Autodesk Inventor part; units mm, degrees
ref_plane "YZ Plane" through (0, 0, 0) normal (1, 0, 0) x (0, 1, 0)
ref_plane "XZ Plane" through (0, 0, 0) normal (0, 1, 0) x (-1, 0, 0)
ref_plane "XY Plane" through (0, 0, 0) normal (0, 0, 1) x (1, 0, 0)
sketch "Sketch1" plane through (0, 0, 0) normal (0, 0, 1) x (1, 0, 0)
  circle A0 centre (0, 0) radius 10
  circle A1 centre (0, 0) radius 8
  dimension "d0" = 20
  dimension "d1" = 2
extrude "Extrusion1" add sketch "Sketch1" along normal blind 115
sketch "Sketch2" plane through (0, 0, 0) normal (0, 0, -1) x (-1, 0, 0)
  circle A0 centre (0, 0) radius 16.5
  circle A1 centre (0, 0) radius 8
  circle A2 centre (0, 0) radius 8 construction
  dimension "d4" = 33
extrude "Extrusion2" add sketch "Sketch2" against normal blind 3
sketch "Sketch3" plane through (0, 0, 3) normal (0, 0, 1) x (1, 0, 0)
  circle A0 centre (9.8995, 9.8995) radius 1.55
  line L0 (9.8995, 9.8995) -> (0, 0) construction
  line L1 (0, 0) -> (4.9931, 0) construction
  dimension "d7" = 14
  dimension "d8" = 3.1
  dimension "d14" = 45
extrude "Extrusion3" cut sketch "Sketch3" against normal through all
sketch "Sketch7" plane through (0, 0, 3) normal (0, 0, 1) x (1, 0, 0)
  circle A0 centre (0, 0) radius 11
  circle A1 centre (0, 0) radius 10
  circle A2 centre (0, 0) radius 10 construction
  dimension "d30" = 1
extrude "Extrusion7" add sketch "Sketch7" along normal blind 2
pattern_circular "Circular Pattern1" count 4 over 360 about axis through (0, 0, 0) along (0, 0, 1) of "Extrusion3"
sketch "Sketch5" plane through (0, 0, 3) normal (0, 0, 1) x (1, 0, 0)
  line L0 (-0.5, 10) -> (0.5, 10)
  line L1 (0.5, 10) -> (0.5, 20)
  line L2 (0.5, 20) -> (-0.5, 20)
  line L3 (-0.5, 20) -> (-0.5, 10)
  line L4 (-0.5, 10) -> (0.5, 20) construction
  line L5 (0.5, 10) -> (-0.5, 20) construction
  point P0 (0, 0)
  point P1 (0, 15)
  point P2 (0, 15)
  dimension "d21" = 1
  dimension "d22" = 10
  dimension "d23" = 10
extrude "Extrusion5" cut sketch "Sketch5" along normal blind 2 and the other way blind 2
sketch "Sketch6" plane through (0, 0, 0) normal (0, 1, 0) x (-1, 0, 0)
  circle A0 centre (0, 112) radius 1.25
  line L0 (10, 115) -> (-10, 115) construction
  point P0 (0, 0)
  dimension "d26" = 3
  dimension "d27" = 2.5
extrude "Extrusion6" cut sketch "Sketch6" along normal through all both and the other way through all
properties part number "Coil_Stand"
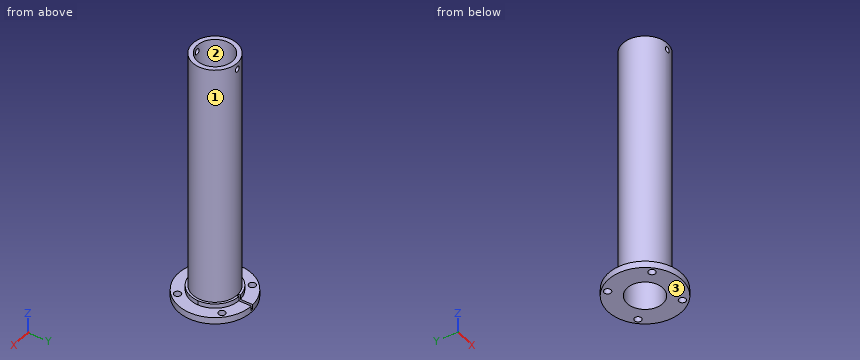
Check sheet for the modelled part. Datum: model origin and axes. Units: mm. Face numbers are marked on the shaded views. Round coordinates to 2 decimals unless told otherwise and drop trailing zeros. Write each loop counter-clockwise with the first axis right and the second up, starting at its lowest first coordinate (ties: lowest second). Pieces come first, ordered by that corner, then holes. Notation, with made-up numbers: (54, 60) -> (81, 60) arc R25 ccw to (81, 74) -> close; hole circle Ø8 at (30, 41). An arc over 180 degrees is marked (long way). Put each result on its own line as item: value.
(1) Sectioned sample at C-C (y = -2). Enter the section's corners in (x, z), plus the area to 3 significant figures.
Values found:
outline: (-16.38, 0) -> (-7.75, 0) -> (-7.75, 115) -> (-9.8, 115) -> (-9.8, 5) -> (-10.82, 5) -> (-10.82, 3) -> (-16.38, 3) -> close; (7.75, 0) -> (16.38, 0) -> (16.38, 3) -> (10.82, 3) -> (10.82, 5) -> (9.8, 5) -> (9.8, 115) -> (7.75, 115) -> close
area: 516 mm^2
(2) Mould release check, pull along Y, two halves, no side actions. Record for the marked faces 1, 2 and 3: released by +Y, released by -Y, zero draft, split by the parting line, or undercut.
Values found:
face 1: split by the parting line
face 2: undercut
face 3: zero draft
(3) Go/stop test with flat-tipped pins: pin 1 Ø3 at (x, z) = (0, 112) entering from -Y; pin 2 Ø10 at (y, z) = (-2, 63.5) entering from +X; pin 3 Ø0.5 at (x, z) = (0, 4) entering from +Y; pin 4 Ø6.5 at (x, y) = (0, 3.5) entering from +Z. Record where each tip stops, or that it passes through.
Values found:
pin 1: stops at y = -10
pin 2: stops at x = 10
pin 3: stops at y = 10
pin 4: passes through
(4) Sectioned sample at A-A (x = -6). Enter the section's corners in (y, z).
Values found:
outline: (-15.37, 0) -> (-5.29, 0) -> (-5.29, 115) -> (-8, 115) -> (-8, 5) -> (-9.22, 5) -> (-9.22, 3) -> (-15.37, 3) -> close; (5.29, 0) -> (15.37, 0) -> (15.37, 3) -> (9.22, 3) -> (9.22, 5) -> (8, 5) -> (8, 115) -> (5.29, 115) -> close
(5) Sectioned sample at B-B (z = 105). Enter the section's corners in (x, y), plus the area to 3 significant figures.
Values found:
outline: circle Ø20 at (0, 0); hole circle Ø16 at (0, 0)
area: 113 mm^2
(6) Material ranges on line 1 (Z direction, x = 0, y = 8.7); line 2 (Z direction, x = 11, y = -1); line 3 (X direction, y = 3, z = 59.5), recorded low to high.
Values found:
line 1: z = 0 to 110.75, 113.25 to 115
line 2: z = 0 to 3
line 3: x = -9.54 to -7.42, 7.42 to 9.54
(7) Sectioned sample at D-D (y = 14). Enter the section's corners in (x, z), plus the area to 3 significant figures.
Values found:
outline: (-8.73, 0) -> (8.73, 0) -> (8.73, 3) -> (0.5, 3) -> (0.5, 1) -> (-0.5, 1) -> (-0.5, 3) -> (-8.73, 3) -> close
area: 50.4 mm^2
